Read the model definition and answer for the solid it produces. Units are mm, in the model's axes. A direction names the side the tool comes from. Coordinates: 2 decimals unless noted, no trailing zeros. Loops run counter-clockwise (first coordinate to the right, second up) from the corner with the lowest first, then second, coordinate; pieces in that order, holes last. Notation, with made-up numbers: M 58.5,36 L 81.5,36 A17 ccw 81.5,50 Z; hole C 29,44.25 d4. An arc over 180 degrees is marked long. Use one line per item in the form item = value. Start each with the question number.
1. The part is cut by section A-A (x = -155.5). Give the vertices of the cut face in (y, z).
2. Find the intervals of material crossed by probe 1 along Y at (x, z) = (-136.5, 1.25); probe 2 along X at (y, z) = (-84.5, 0.2); probe 3 along Y at (x, z) = (-164, 0.6), in increasing order. Write a range as [from, to].
3. A tool of negligible diameter and unlimited length cuts with its end or side. For faces 1 (the flat face through (-125.269, -70, 1)), 2 (the cylindrical face through (-164.699, -75.754, 0.986)), from which of +Z, -Z, +X, -X, +Y, -Y can it reach the whole face along a straight path? Write none if from no direction.
4. For a pull along Y with two mould halves and no side action, classify faces 3 (the flat face through (-150, -65.152, 1)), 4 (the flat face through (-167, -86, 0)), 5 (the flat face through (-165.269, -87, 1)) as released by +Y, released by -Y, zero draft, split by the parting line, or undercut.
5. The part is cut by section C-C (y = -84). Give the vertices of the cut face in (x, z), plus the area to 3 significant figures.
6. The part is cut by section D-D (y = -76.5). Give the vertices of the cut face in (x, z).
7. The part is cut by section B-B (z = 0.55). Give the vertices of the cut face in (x, y).
8. A flat-ended cylindrical pin translates along its axis: pin 1 (1 mm diameter, centred on y = -88, z = 1, fed in from +X). Find the tip coordinate at first contact, or state that the pin passes through.
Autodesk Inventor part; units mm, degrees
ref_plane "YZ Plane" through (0, 0, 0) normal (1, 0, 0) x (0, 1, 0)
ref_plane "XZ Plane" through (0, 0, 0) normal (0, 1, 0) x (-1, 0, 0)
ref_plane "XY Plane" through (0, 0, 0) normal (0, 0, 1) x (1, 0, 0)
sketch "Sketch1" plane through (0, 0, 0) normal (0, 0, 1) x (1, 0, 0)
  circle A0 centre (-170.2692, -86.6522) radius 1.5
  line L0 (-175.2692, -65.1522) -> (-175.2692, -108.1522)
  arc A1 (-163.2692, -75.1522) -> (-165.2692, -77.1522) centre (-163.2692, -77.1522) ccw
  line L1 (-125.2692, -65.1522) -> (-175.2692, -65.1522)
  line L2 (-165.2692, -77.1522) -> (-165.2692, -96.1522)
  line L3 (-125.2692, -75.1522) -> (-125.2692, -65.1522)
  line L4 (-125.2692, -75.1522) -> (-163.2692, -75.1522)
  arc A2 (-165.2692, -96.1522) -> (-163.2692, -98.1522) centre (-163.2692, -96.1522) ccw
  line L5 (-175.2692, -108.1522) -> (-125.2692, -108.1522)
  line L6 (-125.2692, -108.1522) -> (-125.2692, -98.1522)
  line L7 (-163.2692, -98.1522) -> (-125.2692, -98.1522)
  point P0 (0, 0)
  point P1 (-165.2692, -75.1522)
  point P2 (-165.2692, -98.1522)
  dimension "d0" = 40
  dimension "d1" = 23
  dimension "d2" = 2
  dimension "d3" = 10
  dimension "d4" = 50
  dimension "d5" = 43
  dimension "d6" = 3
  dimension "d7" = 5
  dimension "d8" = 21.5
extrude "Extrusion1" add sketch "Sketch1" along normal blind 2
properties part number "cetakan sepatu 2"
Computed values:
q1.outline = M -108.15,0 L -98.15,0 L -98.15,2 L -108.15,2 Z; M -75.15,0 L -65.15,0 L -65.15,2 L -75.15,2 Z
q2.probe_1 = [-108.15, -98.15], [-75.15, -65.15]
q2.probe_2 = [-175.27, -165.27]
q2.probe_3 = [-108.15, -98.01], [-75.29, -65.15]
q3.face_1 = +Z, -Z, +X, +Y, -Y
q3.face_2 = +Z, -Z, +X
q4.face_3 = released by +Y
q4.face_4 = zero draft
q4.face_5 = undercut
q5.outline = M -175.27,0 L -165.27,0 L -165.27,2 L -175.27,2 Z
q5.area = 20.0 mm²
q6.outline = M -175.27,0 L -165.16,0 L -165.16,2 L -175.27,2 Z
q7.outline = M -175.27,-108.15 L -125.27,-108.15 L -125.27,-98.15 L -163.27,-98.15 A2 cw -165.27,-96.15 L -165.27,-77.15 A2 cw -163.27,-75.15 L -125.27,-75.15 L -125.27,-65.15 L -175.27,-65.15 Z; hole C -170.27,-86.65 d3
q8.pin_1 = -165.27
